```python
from build123d import *

# Parameters (mm, degrees)
F0_R     = 25.4
F1_DEPTH = 2.54


with BuildPart() as f1:
    # F0 (on Top) → F1 (new body)
    with BuildSketch(Plane.XY):
        Circle(F0_R)
        with BuildLine():
            Line((-16.63807, -7.666502), (-8.386692, -8.386692))
            Line((-8.386692, -8.386692), (-7.666502, -16.63807))
            Line((-7.666502, -16.63807), (-11.43, -19.797341))
            ThreePointArc((-11.43, -19.797341), (-16.164461, -16.164461), (-19.797341, -11.43))
            Line((-19.797341, -11.43), (-16.63807, -7.666502))
        make_face(mode=Mode.SUBTRACT)
        with BuildLine():
            ThreePointArc((-7.225741, -21.687975), (-8.748143, -21.119886), (-10.226344, -20.445085))
            Line((-10.226344, -20.445085), (-7.531657, -18.183027))
            Line((-7.531657, -18.183027), (-7.225741, -21.687975))
        make_face(mode=Mode.SUBTRACT)
        with BuildLine():
            Line((-6.343856, -17.185928), (0, -11.860573))
            Line((0, -11.860573), (6.343856, -17.185928))
            Line((6.343856, -17.185928), (5.916603, -22.081064))
            ThreePointArc((5.916603, -22.081064), (0, -22.86), (-5.916603, -22.081064))
            Line((-5.916603, -22.081064), (-6.343856, -17.185928))
        make_face(mode=Mode.SUBTRACT)
        with BuildLine():
            Line((-21.687975, -7.225741), (-18.183027, -7.531657))
            Line((-18.183027, -7.531657), (-20.445085, -10.226344))
            ThreePointArc((-20.445085, -10.226344), (-21.119886, -8.748143), (-21.687975, -7.225741))
        make_face(mode=Mode.SUBTRACT)
        with BuildLine():
            Line((-7.142111, -8.040137), (-6.282752, -7.180777))
            Line((-6.282752, -7.180777), (-3.923092, -7.096107))
            ThreePointArc((-3.923092, -7.096107), (-3.102932, -7.491142), (-2.243661, -7.791751))
            Line((-2.243661, -7.791751), (-0.635, -9.520153))
            Line((-0.635, -9.520153), (-0.635, -10.73547))
            Line((-0.635, -10.73547), (-6.478702, -15.64097))
            Line((-6.478702, -15.64097), (-7.142111, -8.040137))
        make_face(mode=Mode.SUBTRACT)
        with BuildLine():
            Line((-10.73547, -0.635), (-9.520153, -0.635))
            Line((-9.520153, -0.635), (-7.791751, -2.243661))
            ThreePointArc((-7.791751, -2.243661), (-7.491142, -3.102932), (-7.096107, -3.923092))
            Line((-7.096107, -3.923092), (-7.180777, -6.282752))
            Line((-7.180777, -6.282752), (-8.040137, -7.142111))
            Line((-8.040137, -7.142111), (-15.64097, -6.478702))
            Line((-15.64097, -6.478702), (-10.73547, -0.635))
        make_face(mode=Mode.SUBTRACT)
        with BuildLine():
            Line((-6.474615, -2.200555), (-1.803671, -0.613021))
            ThreePointArc((-1.803671, -0.613021), (-1.347038, -1.347038), (-0.613021, -1.803671))
            Line((-0.613021, -1.803671), (-2.200555, -6.474615))
            ThreePointArc((-2.200555, -6.474615), (-4.835446, -4.835446), (-6.474615, -2.200555))
        make_face(mode=Mode.SUBTRACT)
        with BuildLine():
            ThreePointArc((10.226344, -20.445085), (8.748143, -21.119886), (7.225741, -21.687975))
            Line((7.225741, -21.687975), (7.531657, -18.183027))
            Line((7.531657, -18.183027), (10.226344, -20.445085))
        make_face(mode=Mode.SUBTRACT)
        with BuildLine():
            Line((7.666502, -16.63807), (8.386692, -8.386692))
            Line((8.386692, -8.386692), (16.63807, -7.666502))
            Line((16.63807, -7.666502), (19.797341, -11.43))
            ThreePointArc((19.797341, -11.43), (16.164461, -16.164461), (11.43, -19.797341))
            Line((11.43, -19.797341), (7.666502, -16.63807))
        make_face(mode=Mode.SUBTRACT)
        with BuildLine():
            Line((0.635, -10.73547), (0.635, -9.520153))
            Line((0.635, -9.520153), (2.243661, -7.791751))
            ThreePointArc((2.243661, -7.791751), (3.102932, -7.491142), (3.923092, -7.096107))
            Line((3.923092, -7.096107), (6.282752, -7.180777))
            Line((6.282752, -7.180777), (7.142111, -8.040137))
            Line((7.142111, -8.040137), (6.478702, -15.64097))
            Line((6.478702, -15.64097), (0.635, -10.73547))
        make_face(mode=Mode.SUBTRACT)
        with BuildLine():
            Line((2.200555, -6.474615), (0.613021, -1.803671))
            ThreePointArc((0.613021, -1.803671), (1.347038, -1.347038), (1.803671, -0.613021))
            Line((1.803671, -0.613021), (6.474615, -2.200555))
            ThreePointArc((6.474615, -2.200555), (4.835446, -4.835446), (2.200555, -6.474615))
        make_face(mode=Mode.SUBTRACT)
        with BuildLine():
            Line((8.040137, -7.142111), (7.180777, -6.282752))
            Line((7.180777, -6.282752), (7.096107, -3.923092))
            ThreePointArc((7.096107, -3.923092), (7.491142, -3.102932), (7.791751, -2.243661))
            Line((7.791751, -2.243661), (9.520153, -0.635))
            Line((9.520153, -0.635), (10.73547, -0.635))
            Line((10.73547, -0.635), (15.64097, -6.478702))
            Line((15.64097, -6.478702), (8.040137, -7.142111))
        make_face(mode=Mode.SUBTRACT)
        with BuildLine():
            ThreePointArc((21.687975, -7.225741), (21.119886, -8.748143), (20.445085, -10.226344))
            Line((20.445085, -10.226344), (18.183027, -7.531657))
            Line((18.183027, -7.531657), (21.687975, -7.225741))
        make_face(mode=Mode.SUBTRACT)
        with BuildLine():
            Line((17.185928, -6.343856), (11.860573, 0))
            Line((11.860573, 0), (17.185928, 6.343856))
            Line((17.185928, 6.343856), (22.081064, 5.916603))
            ThreePointArc((22.081064, 5.916603), (22.86, 0), (22.081064, -5.916603))
            Line((22.081064, -5.916603), (17.185928, -6.343856))
        make_face(mode=Mode.SUBTRACT)
        with BuildLine():
            Line((-17.185928, 6.343856), (-11.860573, 0))
            Line((-11.860573, 0), (-17.185928, -6.343856))
            Line((-17.185928, -6.343856), (-22.081064, -5.916603))
            ThreePointArc((-22.081064, -5.916603), (-22.86, 0), (-22.081064, 5.916603))
            Line((-22.081064, 5.916603), (-17.185928, 6.343856))
        make_face(mode=Mode.SUBTRACT)
        with BuildLine():
            Line((-20.445085, 10.226344), (-18.183027, 7.531657))
            Line((-18.183027, 7.531657), (-21.687975, 7.225741))
            ThreePointArc((-21.687975, 7.225741), (-21.119886, 8.748143), (-20.445085, 10.226344))
        make_face(mode=Mode.SUBTRACT)
        with BuildLine():
            Line((-8.040137, 7.142111), (-7.180777, 6.282752))
            Line((-7.180777, 6.282752), (-7.096107, 3.923092))
            ThreePointArc((-7.096107, 3.923092), (-7.491142, 3.102932), (-7.791751, 2.243661))
            Line((-7.791751, 2.243661), (-9.520153, 0.635))
            Line((-9.520153, 0.635), (-10.73547, 0.635))
            Line((-10.73547, 0.635), (-15.64097, 6.478702))
            Line((-15.64097, 6.478702), (-8.040137, 7.142111))
        make_face(mode=Mode.SUBTRACT)
        with BuildLine():
            Line((-2.200555, 6.474615), (-0.613021, 1.803671))
            ThreePointArc((-0.613021, 1.803671), (-1.347038, 1.347038), (-1.803671, 0.613021))
            Line((-1.803671, 0.613021), (-6.474615, 2.200555))
            ThreePointArc((-6.474615, 2.200555), (-4.835446, 4.835446), (-2.200555, 6.474615))
        make_face(mode=Mode.SUBTRACT)
        with BuildLine():
            Line((-0.635, 10.73547), (-0.635, 9.520153))
            Line((-0.635, 9.520153), (-2.243661, 7.791751))
            ThreePointArc((-2.243661, 7.791751), (-3.102932, 7.491142), (-3.923092, 7.096107))
            Line((-3.923092, 7.096107), (-6.282752, 7.180777))
            Line((-6.282752, 7.180777), (-7.142111, 8.040137))
            Line((-7.142111, 8.040137), (-6.478702, 15.64097))
            Line((-6.478702, 15.64097), (-0.635, 10.73547))
        make_face(mode=Mode.SUBTRACT)
        with BuildLine():
            ThreePointArc((-19.797341, 11.43), (-16.164461, 16.164461), (-11.43, 19.797341))
            Line((-11.43, 19.797341), (-7.666502, 16.63807))
            Line((-7.666502, 16.63807), (-8.386692, 8.386692))
            Line((-8.386692, 8.386692), (-16.63807, 7.666502))
            Line((-16.63807, 7.666502), (-19.797341, 11.43))
        make_face(mode=Mode.SUBTRACT)
        with BuildLine():
            Line((-7.225741, 21.687975), (-7.531657, 18.183027))
            Line((-7.531657, 18.183027), (-10.226344, 20.445085))
            ThreePointArc((-10.226344, 20.445085), (-8.748143, 21.119886), (-7.225741, 21.687975))
        make_face(mode=Mode.SUBTRACT)
        with BuildLine():
            ThreePointArc((1.803671, 0.613021), (1.347038, 1.347038), (0.613021, 1.803671))
            Line((0.613021, 1.803671), (2.200555, 6.474615))
            ThreePointArc((2.200555, 6.474615), (4.835446, 4.835446), (6.474615, 2.200555))
            Line((6.474615, 2.200555), (1.803671, 0.613021))
        make_face(mode=Mode.SUBTRACT)
        with BuildLine():
            Line((10.73547, 0.635), (9.520153, 0.635))
            Line((9.520153, 0.635), (7.791751, 2.243661))
            ThreePointArc((7.791751, 2.243661), (7.491142, 3.102932), (7.096107, 3.923092))
            Line((7.096107, 3.923092), (7.180777, 6.282752))
            Line((7.180777, 6.282752), (8.040137, 7.142111))
            Line((8.040137, 7.142111), (15.64097, 6.478702))
            Line((15.64097, 6.478702), (10.73547, 0.635))
        make_face(mode=Mode.SUBTRACT)
        with BuildLine():
            Line((2.243661, 7.791751), (0.635, 9.520153))
            Line((0.635, 9.520153), (0.635, 10.73547))
            Line((0.635, 10.73547), (6.478702, 15.64097))
            Line((6.478702, 15.64097), (7.142111, 8.040137))
            Line((7.142111, 8.040137), (6.282752, 7.180777))
            Line((6.282752, 7.180777), (3.923092, 7.096107))
            ThreePointArc((3.923092, 7.096107), (3.102932, 7.491142), (2.243661, 7.791751))
        make_face(mode=Mode.SUBTRACT)
        with BuildLine():
            ThreePointArc((20.445085, 10.226344), (21.119886, 8.748143), (21.687975, 7.225741))
            Line((21.687975, 7.225741), (18.183027, 7.531657))
            Line((18.183027, 7.531657), (20.445085, 10.226344))
        make_face(mode=Mode.SUBTRACT)
        with BuildLine():
            Line((6.343856, 17.185928), (0, 11.860573))
            Line((0, 11.860573), (-6.343856, 17.185928))
            Line((-6.343856, 17.185928), (-5.916603, 22.081064))
            ThreePointArc((-5.916603, 22.081064), (0, 22.86), (5.916603, 22.081064))
            Line((5.916603, 22.081064), (6.343856, 17.185928))
        make_face(mode=Mode.SUBTRACT)
        with BuildLine():
            ThreePointArc((7.225741, 21.687975), (8.748143, 21.119886), (10.226344, 20.445085))
            Line((10.226344, 20.445085), (7.531657, 18.183027))
            Line((7.531657, 18.183027), (7.225741, 21.687975))
        make_face(mode=Mode.SUBTRACT)
        with BuildLine():
            Line((16.63807, 7.666502), (8.386692, 8.386692))
            Line((8.386692, 8.386692), (7.666502, 16.63807))
            Line((7.666502, 16.63807), (11.43, 19.797341))
            ThreePointArc((11.43, 19.797341), (16.164461, 16.164461), (19.797341, 11.43))
            Line((19.797341, 11.43), (16.63807, 7.666502))
        make_face(mode=Mode.SUBTRACT)
    extrude(amount=F1_DEPTH)


solid = f1.part
```
The model under review builds one solid part; all positions refer to its coordinate system, in mm. Round coordinates to 2 decimals unless told otherwise and drop trailing zeros. Write each loop counter-clockwise with the first axis right and the second up, starting at its lowest first coordinate (ties: lowest second). Pieces come first, ordered by that corner, then holes. Notation, with made-up numbers: M -20,8 L 22,8 A17 ccw 22,36 Z; hole C 30.25,-20 d9. An arc over 180 degrees is marked long. Use CSV: the item, a comma, the result in double quotes. Start each with the question number.
(1) We need section B-B, the plane z = 1.3. State how many separate pieces and enclosed holes the cut face has, then the cut area to 3 significant figures.
(2) For line 1 along X through (y, z) = (-17.5, 2.35); line 2 along Y through (x, z) = (0.5, 1.25); line 3 along X through (y, z) = (-10.5, 0.3) (3 decimals), list the stretches that pass through material, from the lowest coordinate up.
(3) We need section A-A, the plane x = 14. State the section outline as (y, z) points, then the cut area to 3 significant figures.
(4) Clearance check with flat-ended pins moving along their axes: P1, Ø1.5, axis at x = 8, z = 1.5, coming from the +Y side; P2, Ø1.3, axis at x = 10, z = 0.5, coming from the -Y side; P3, Ø1, axis at x = -10, z = 1, coming from the +Y side; P4, Ø8, axis at x = 11.5, y = -12.5, coming from the +Z side. State where each tip first meets the part, or that it passes through.
Findings:
1,separate pieces,"1"
1,enclosed holes,"28"
1,area,"826 mm^2"
2,line 1,"-18.41 to -14.71, -8.69 to -6.32, 6.32 to 8.69, 14.71 to 18.41"
2,line 2,"-25.4 to -22.85, -12.28 to 12.28, 22.85 to 25.4"
2,line 3,"-23.128 to -19.017, -8.202 to -6.927, -0.635 to 0.635, 6.927 to 8.202, 19.017 to 23.128"
3,outline,"M -21.19,0 L -18.07,0 L -18.07,2.54 L -21.19,2.54 Z; M -7.9,0 L -6.62,0 L -6.62,2.54 L -7.9,2.54 Z; M -4.52,0 L -2.55,0 L -2.55,2.54 L -4.52,2.54 Z; M 2.55,0 L 4.52,0 L 4.52,2.54 L 2.55,2.54 Z; M 6.62,0 L 7.9,0 L 7.9,2.54 L 6.62,2.54 Z; M 18.07,0 L 21.19,0 L 21.19,2.54 L 18.07,2.54 Z"
3,area,"32.4 mm^2"
4,P1,"y = 24.34"
4,P2,"y = -23.62"
4,P3,"y = 23.56"
4,P4,"z = 2.54"
